Verification items for the finished model (mm, model axes). A direction names the side the tool comes from. Coordinates: 2 decimals unless noted, no trailing zeros. Order: outer loops, then holes, each group sorted by start corner. A loop starts at its lowest first (then second) coordinate and runs counter-clockwise, first axis right, second up. Notation, with made-up numbers: M -0.5,-13.5 L 19.5,-13.5 A17 ccw 19.5,-9.5 Z; hole C 28.5,15.25 d2. An arc over 180 degrees is marked long. Return JSON: item names as keys, results as strings. Group by question number.
Q1. Section check B-B, the plane x = -4.5. Enter the section's corners in (y, z).
Q2. Section check C-C, the plane x = -43. Enter the section's corners in (y, z), then the cut area to 3 significant figures.
Q3. Go/stop test with flat-tipped pins: pin 1 Ø8 at (x, y) = (21.5, 8.5) entering from +Z; pin 2 Ø4 at (x, y) = (-17.5, 11) entering from +Z; pin 3 Ø4 at (x, z) = (3, 130.5) entering from -Y; pin 4 Ø8 at (x, y) = (6.5, 3.5) entering from -Z. Record where each tip stops, or that it passes through.
Q4. Section check D-D, the plane z = 63.5. Enter the section's corners in (x, y), then the cut area to 3 significant figures.
Q5. Section check A-A, the plane z = 0. Enter the section's corners in (x, y), then the cut area to 3 significant figures.
Q6. Mould release check, pull along Z, two halves, no side actions. Record for faces 1 (the face through (-21, 16, 92)), 2 (the face through (-34.116, 7.888, 188.937)), 3 (the face through (25.18, 7.89, 196.31)): pulls with the +Z half, pulls with the -Z half, needs draft (parallel to the pull), parting line crosses it, or undercut.
Q7. Access from +Z, -Z, +X, -X, +Y, -Y to the whole of each face (thin tool, end or side, straight path). Record for faces 4 (the face through (-43.86, 7, 153.17)), 5 (the face through (24, 8, -18)), 6 (the face through (3.54, 8.11, 35.15)).
Q8. Thickness scan on probe 1 along Z at (x, y) = (-4, 7); probe 2 along Z at (x, y) = (-43.25, 8); probe 3 along Z at (x, y) = (10, 9.5). Record the ranges inside material, lowest first.
Autodesk Inventor part; units mm, degrees
ref_plane "YZ Plane" through (0, 0, 0) normal (1, 0, 0) x (0, 1, 0)
ref_plane "XZ Plane" through (0, 0, 0) normal (0, 1, 0) x (-1, 0, 0)
ref_plane "XY Plane" through (0, 0, 0) normal (0, 0, 1) x (1, 0, 0)
sketch "Sketch1" plane through (0, 0, 0) normal (0, 1, 0) x (-1, 0, 0)
  arc A0 (0, 30) -> (20.6897, -21.7241) centre (0, 0) ccw
  arc A1 (20.6897, 201.7241) -> (0, 150) centre (0, 180) ccw
  line L0 (54, 10) -> (54, 170)
  line L1 (0, 150) -> (0, 30)
  line L2 (54, 10) -> (20.6897, -21.7241)
  line L3 (54, 170) -> (20.6897, 201.7241)
extrude "Extrusion2" add sketch "Sketch1" along normal blind 16
hole "Hole3" at (0, 0, 180) at (0, 0, 0) direction (0, 1, 0) diameter 42 depth 16
fillet "Fillet3" radius 22 2 edges at (0, 8, 30) (0, 8, 150)
sketch "Sketch4" plane through (-54, 0, 10) normal (-1, 0, 0) x (0, 0, 1)
  line L0 (0, 0) -> (0, 16)
  line L1 (0, 8) -> (160, 8)
  line L2 (160, 0) -> (160, 16)
  point P0 (-10, 0)
  point P1 (20, 8)
  point P2 (140, 8)
fillet "Fillet4" radius 22 2 edges at (-54, 8, 10) (-54, 8, 170)
hole "Hole4" at (-54, 8, 30) at (-54, 8, 150) direction (1, 0, 0) diameter 6.647 depth 20 tip angle 118
properties part number "TelescopeMountConnector"
Numbers:
{
 "1": {"outline": "M 0,-29.66 L 16,-29.66 L 16,-20.51 L 0,-20.51 Z; M 0,20.51 L 16,20.51 L 16,159.49 L 0,159.49 Z; M 0,200.51 L 16,200.51 L 16,209.66 L 0,209.66 Z"},
 "2": {"outline": "M 0,-0.48 L 16,-0.48 L 16,180.48 L 0,180.48 Z; hole C 8,30 d6.65; hole C 8,150 d6.65", "area": "2,830 mm2"},
 "3": {"pin 1": "stops at z = 204.37", "pin 2": "stops at z = 205.69", "pin 3": "passes through", "pin 4": "stops at z = -29.9"},
 "4": {"outline": "M -54,0 L 0,0 L 0,16 L -54,16 Z", "area": "864 mm2"},
 "5": {"outline": "M -43.5,0 L -21,0 L -21,16 L -43.5,16 Z; M 21,0 L 30,0 L 30,16 L 21,16 Z", "area": "504 mm2"},
 "6": {"face 1": "needs draft", "face 2": "pulls with the +Z half", "face 3": "undercut"},
 "7": {"face 4": "-X", "face 5": "+Y, -Y", "face 6": "+X, +Y, -Y"},
 "8": {"probe 1": "z = -29.73 to -20.62, 20.62 to 159.38, 200.62 to 209.73", "probe 2": "z = -0.24 to 26.68, 33.32 to 146.68, 153.32 to 180.24", "probe 3": "z = -28.28 to -18.47, 18.47 to 28.68, 151.32 to 161.53, 198.47 to 208.28"}
}
